Geometry check sheet. Reference: the model listing, model coordinates, mm. Face numbers are marked on the shaded views. Round coordinates to 2 decimals unless told otherwise and drop trailing zeros. Loops run counter-clockwise (first coordinate to the right, second up) from the corner with the lowest first, then second, coordinate; pieces in that order, holes last.
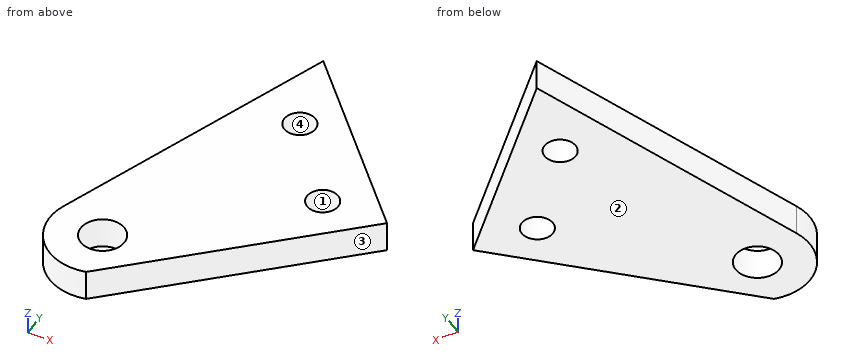
```python
from build123d import *

# Parameters (mm, degrees)
SKETCH1_R           = 1.5
BOSS_EXTRUDE1_DEPTH = 3
SKETCH3_R           = 2.1
CUT_EXTRUDE1_DEPTH  = 5
BOSS_EXTRUDE2_START = -3
SKETCH4_R           = 2.1
SKETCH4_R_2         = 1.5
BOSS_EXTRUDE2_DEPTH = 3


with BuildPart() as part:
    # Sketch1 → Boss-Extrude1 (new body)
    with BuildSketch(Plane.XY):
        with BuildLine():
            Line((-23.846751299, 12.315625527), (-25.790964416, 1.588420048))
            ThreePointArc((-25.790964416, 1.588420048), (-23.621324023, -2.99099118), (-18.587504633, -2.408746401))
            Line((-18.587504633, -2.408746401), (-9.554934768, 5.787656918))
            Line((-9.554934768, 5.787656918), (-6.092344559, 8.929706888))
            Line((-6.092344559, 8.929706888), (-21.437418033, 24.964674832))
            Line((-21.437418033, 24.964674832), (-22.045496957, 21.772247946))
            Line((-22.045496957, 21.772247946), (-23.846751299, 12.315625527))
        make_face()
        with Locations((-19.053986742, 16.730936194)):
            Circle(SKETCH1_R, mode=Mode.SUBTRACT)
        with Locations((-12.303254046, 8.7654358)):
            Circle(SKETCH1_R, mode=Mode.SUBTRACT)
    extrude(amount=BOSS_EXTRUDE1_DEPTH)

    # Sketch3 → Cut-Extrude1 (cut)
    with BuildSketch(Plane.XY.offset(3)):
        with Locations((-21.51274635, 0.809673644)):
            Circle(SKETCH3_R)
    extrude(amount=-CUT_EXTRUDE1_DEPTH, mode=Mode.SUBTRACT)

    # Sketch4 → Boss-Extrude2 (add)
    with BuildSketch(Plane.XY.offset(3).offset(BOSS_EXTRUDE2_START)):
        with BuildLine():
            Line((-21.437418033, 24.964674832), (-6.092344559, 8.929706888))
            Line((-6.092344559, 8.929706888), (-25.203805177, -9.359495085))
            ThreePointArc((-25.203805177, -9.359495085), (-30.162494982, -7.817509351), (-31.18157458, -2.725574419))
            Line((-31.18157458, -2.725574419), (-21.437418033, 24.964674832))
        make_face()
        with Locations((-26.38487303, -4.41352639)):
            Circle(SKETCH4_R, mode=Mode.SUBTRACT)
        with Locations((-12.303254046, 8.7654358)):
            Circle(SKETCH4_R_2, mode=Mode.SUBTRACT)
        with Locations((-19.053986742, 16.730936194)):
            Circle(SKETCH4_R_2, mode=Mode.SUBTRACT)
    extrude(amount=BOSS_EXTRUDE2_DEPTH)


solid = part.part
```
1) Sectioned sample at C-C, the plane x = -27.5. Record the cut outline in (y, z), then the cut area to 3 significant figures.
Report:
outline: (-9.37, 0) - (-6.19, 0) - (-6.19, 3) - (-9.37, 3) - close; (-2.63, 0) - (7.74, 0) - (7.74, 3) - (-2.63, 3) - close
area: 40.7 mm2
2) Mould release check, pull along X, two halves, no side actions. Record for the marked faces 1, 2, 3 and 4: +X half, -X half, draft (parallel to the pull), parting line (faces both ways), or undercut.
Report:
face 1: undercut
face 2: draft
face 3: +X half
face 4: undercut
3) Sectioned sample at B-B, the plane z = 1.1. Record the cut outline in (x, y), then the cut area to 3 significant figures.
Report:
outline: (-31.18, -2.73) arc R5.09 ccw to (-25.2, -9.36) - (-6.09, 8.93) - (-21.44, 24.96) - close; hole circle Ø4.2 at (-26.38, -4.41); hole circle Ø3 at (-19.05, 16.73); hole circle Ø3 at (-12.3, 8.77)
area: 397 mm2
4) Scan lines: line 1 along Y through (x, z) = (-11.25, 1.7); line 2 along X through (y, z) = (8, 1.2); line 3 along X through (y, z) = (-5, 2.9). Record each from-to range of solid material in increasing order.
Report:
line 1: y = 3.99 to 7.7, 9.83 to 14.32
line 2: x = -27.41 to -13.59, -11.01 to -7.06
line 3: x = -31.44 to -28.4, -24.37 to -20.65
5) Sectioned sample at D-D, the plane y = 4.5. Record the cut outline in (x, z), then the cut area to 3 significant figures.
Report:
outline: (-28.64, 0) - (-10.72, 0) - (-10.72, 3) - (-28.64, 3) - close
area: 53.8 mm2
6) Sectioned sample at A-A, the plane x = -11.5. Record the cut outline in (y, z).
Report:
outline: (3.75, 0) - (7.5, 0) - (7.5, 3) - (3.75, 3) - close; (10.03, 0) - (14.58, 0) - (14.58, 3) - (10.03, 3) - close
